Can you work these out from the model? Positions are in its coordinate system, mm. Face numbers are marked on the shaded views. A direction names the side the tool comes from. Coordinates: 2 decimals unless noted, no trailing zeros. Order: outer loops, then holes, each group sorted by start corner. A loop starts at its lowest first (then second) coordinate and runs counter-clockwise, first axis right, second up. Notation, with made-up numbers: (17.5, 5) -> (72.5, 5) arc R8 ccw to (72.5, 12) -> close; hole circle Ø10 at (-17.5, 49). An arc over 180 degrees is marked (long way). Answer as a JSON object with one key per item and string values. Group by question number.
(1) For pin 1 (1.1 mm diameter, centred on y = 14, z = 1, fed in from +X); pin 2 (1.1 mm diameter, centred on x = -1, z = 1.5, fed in from +Y); pin 3 (0.7 mm diameter, centred on x = 3, z = 1, fed in from -Y), each with a flat end and sliding along its axis, tell me the tip position at first contact or that it passes through.
(2) I want a section at A-A, the plane y = 6.75. List the corners of the cut face in (x, z) for me.
(3) I want a section at D-D, the plane y = 15.25. List the corners of the cut face in (x, z) for me.
(4) I want a section at C-C, the plane z = 0.45. State how many separate pieces and enclosed holes the cut face has, plus the area to 3 significant figures.
(5) Which directions (+Z, -Z, +X, -X, +Y, -Y) give clear straight access to the entire face, cutting with the end or side of a thin tool? Please do the marked faces 1, 2, 3, 4 and 5.
(6) If we mould it in two halves opening along Y, with no side actions, what happens to the marked faces 6, 7 and 8? For each: pulls with the +Y half, pulls with the -Y half, needs draft (parallel to the pull), parting line crosses it, or undercut.
(7) I need wall thicknesses on line 1 (X direction, y = 5.75, z = 1.1); line 2 (Y direction, x = 6, z = 1.3); line 3 (X direction, y = 1.5, z = 0.95). Which ranges of each line are inside material? Lowest first, please.
(8) I want a section at B-B, the plane x = 10.5. List the corners of the cut face in (y, z) for me, plus the area to 3 significant figures.
from build123d import *

# Parameters (mm, degrees)
F0_W     = 3
F0_H     = 3
F1_DEPTH = 2.2


with BuildPart() as f1:
    # F0 (on Top) → F1 (new body)
    with BuildSketch(Plane.XY):
        with BuildLine():
            Line((1, 3), (4, 3))
            Line((4, 3), (4, 0.854192))
            ThreePointArc((4, 0.854192), (4.496745, 0.725778), (5, 0.62588))
            Line((5, 0.62588), (5, 3))
            Line((5, 3), (8, 3))
            Line((8, 3), (8, 0.62588))
            ThreePointArc((8, 0.62588), (8.503255, 0.725778), (9, 0.854192))
            Line((9, 0.854192), (9, 3))
            Line((9, 3), (12, 3))
            Line((12, 3), (12, 2.376097))
            ThreePointArc((12, 2.376097), (12.863961, 3.136039), (13.623903, 4))
            Line((13.623903, 4), (13, 4))
            Line((13, 4), (13, 7))
            Line((13, 7), (15.145808, 7))
            ThreePointArc((15.145808, 7), (15.274222, 7.496745), (15.37412, 8))
            Line((15.37412, 8), (13, 8))
            Line((13, 8), (13, 11))
            Line((13, 11), (15.37412, 11))
            ThreePointArc((15.37412, 11), (15.274222, 11.503255), (15.145808, 12))
            Line((15.145808, 12), (13, 12))
            Line((13, 12), (13, 15))
            Line((13, 15), (13.623903, 15))
            ThreePointArc((13.623903, 15), (12.863961, 15.863961), (12, 16.623903))
            Line((12, 16.623903), (12, 16))
            Line((12, 16), (9, 16))
            Line((9, 16), (9, 18.145808))
            ThreePointArc((9, 18.145808), (8.503255, 18.274222), (8, 18.37412))
            Line((8, 18.37412), (8, 16))
            Line((8, 16), (5, 16))
            Line((5, 16), (5, 18.37412))
            ThreePointArc((5, 18.37412), (4.496745, 18.274222), (4, 18.145808))
            Line((4, 18.145808), (4, 16))
            Line((4, 16), (1, 16))
            Line((1, 16), (1, 16.623903))
            ThreePointArc((1, 16.623903), (0.136039, 15.863961), (-0.623903, 15))
            Line((-0.623903, 15), (0, 15))
            Line((0, 15), (0, 12))
            Line((0, 12), (-2.145808, 12))
            ThreePointArc((-2.145808, 12), (-2.274222, 11.503255), (-2.37412, 11))
            Line((-2.37412, 11), (0, 11))
            Line((0, 11), (0, 8))
            Line((0, 8), (-2.37412, 8))
            ThreePointArc((-2.37412, 8), (-2.274222, 7.496745), (-2.145808, 7))
            Line((-2.145808, 7), (0, 7))
            Line((0, 7), (0, 4))
            Line((0, 4), (-0.623903, 4))
            ThreePointArc((-0.623903, 4), (0.136039, 3.136039), (1, 2.376097))
            Line((1, 2.376097), (1, 3))
        make_face()
        with Locations((2.5, 5.5)):
            Rectangle(F0_W, F0_H, mode=Mode.SUBTRACT)
        with Locations((6.5, 5.5)):
            Rectangle(F0_W, F0_H, mode=Mode.SUBTRACT)
        with Locations((10.5, 5.5)):
            Rectangle(F0_W, F0_H, mode=Mode.SUBTRACT)
        with Locations((2.5, 9.5)):
            Rectangle(F0_W, F0_H, mode=Mode.SUBTRACT)
        with Locations((2.5, 13.5)):
            Rectangle(F0_W, F0_H, mode=Mode.SUBTRACT)
        with Locations((6.5, 9.5)):
            Rectangle(F0_W, F0_H, mode=Mode.SUBTRACT)
        with Locations((10.5, 9.5)):
            Rectangle(F0_W, F0_H, mode=Mode.SUBTRACT)
        with Locations((6.5, 13.5)):
            Rectangle(F0_W, F0_H, mode=Mode.SUBTRACT)
        with Locations((10.5, 13.5)):
            Rectangle(F0_W, F0_H, mode=Mode.SUBTRACT)
    extrude(amount=F1_DEPTH)


solid = f1.part
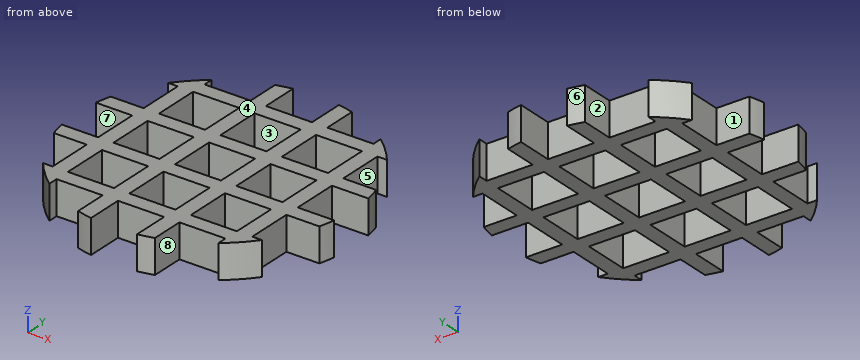
Computed values:
{
 "1": {"pin 1": "stops at x = 13", "pin 2": "stops at y = 15.22", "pin 3": "stops at y = 3"},
 "2": {"outline": "(0, 0) -> (1, 0) -> (1, 2.2) -> (0, 2.2) -> close; (4, 0) -> (5, 0) -> (5, 2.2) -> (4, 2.2) -> close; (8, 0) -> (9, 0) -> (9, 2.2) -> (8, 2.2) -> close; (12, 0) -> (13, 0) -> (13, 2.2) -> (12, 2.2) -> close"},
 "3": {"outline": "(-0.42, 0) -> (13.42, 0) -> (13.42, 2.2) -> (-0.42, 2.2) -> close"},
 "4": {"separate pieces": "1", "enclosed holes": "9", "area": "108 mm2"},
 "5": {"face 1": "+Z, -Z, -X", "face 2": "+Z, -Z, +Y", "face 3": "+Z, -Z", "face 4": "+Z, +X, -X, +Y, -Y", "face 5": "+Z, -Z, +X"},
 "6": {"face 6": "pulls with the +Y half", "face 7": "undercut", "face 8": "needs draft"},
 "7": {"line 1": "x = 0 to 1, 4 to 5, 8 to 9, 12 to 13", "line 2": "y = 3 to 4, 7 to 8, 11 to 12, 15 to 16", "line 3": "x = 4 to 5, 8 to 9"},
 "8": {"outline": "(3, 0) -> (4, 0) -> (4, 2.2) -> (3, 2.2) -> close; (7, 0) -> (8, 0) -> (8, 2.2) -> (7, 2.2) -> close; (11, 0) -> (12, 0) -> (12, 2.2) -> (11, 2.2) -> close; (15, 0) -> (16, 0) -> (16, 2.2) -> (15, 2.2) -> close", "area": "8.80 mm2"}
}
